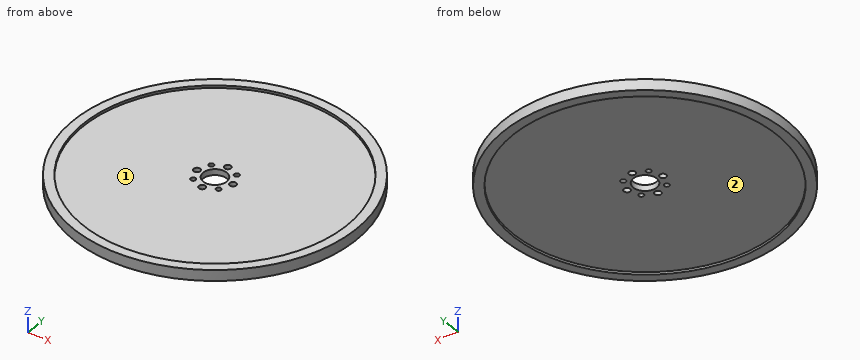
from build123d import *

# Parameters (mm, degrees)
SKETCH1_R                 = 76.2
SKETCH1_R_2               = 71.12
BOSS_EXTRUDE1_DEPTH       = 2.921
SKETCH3_R                 = 71.12
SKETCH3_R_2               = 6.35
SKETCH3_R_3               = 1.778
BOSS_EXTRUDE2_DEPTH       = 1.5875
F_6_32_TAPPED_HOLE1_D     = 2.7051
F_6_32_TAPPED_HOLE1_DEPTH = 3.175


with BuildPart() as part:
    # Sketch1 → Boss-Extrude1 (new body, symmetric)
    with BuildSketch(Plane.XY):
        Circle(SKETCH1_R)
        Circle(SKETCH1_R_2, mode=Mode.SUBTRACT)
    extrude(amount=BOSS_EXTRUDE1_DEPTH, both=True)

    # Sketch3 → Boss-Extrude2 (add, symmetric)
    with BuildSketch(Plane.XY):
        Circle(SKETCH3_R)
        Circle(SKETCH3_R_2, mode=Mode.SUBTRACT)
        with Locations((0, 9.779)):
            Circle(SKETCH3_R_3, mode=Mode.SUBTRACT)
        with Locations((9.779, 0)):
            Circle(SKETCH3_R_3, mode=Mode.SUBTRACT)
        with Locations((0, -9.779)):
            Circle(SKETCH3_R_3, mode=Mode.SUBTRACT)
        with Locations((-9.779, 0)):
            Circle(SKETCH3_R_3, mode=Mode.SUBTRACT)
    extrude(amount=BOSS_EXTRUDE2_DEPTH, both=True)

    # #6-32 Tapped Hole1
    with Locations(Plane.XY.offset(1.5875)):
        with Locations((-6.914797213, 6.914797213), (6.914797213, 6.914797213), (6.914797213, -6.914797213), (-6.914797213, -6.914797213)):
            Hole(F_6_32_TAPPED_HOLE1_D / 2, depth=F_6_32_TAPPED_HOLE1_DEPTH)


solid = part.part
For this review, take the finished solid that the model builds, in its own axes (mm). Face numbers are marked on the shaded views. A direction names the side the tool comes from. Give positions to 0.01 mm unless a question says otherwise; leave off trailing zeros. Loops run counter-clockwise (first coordinate to the right, second up) from the corner with the lowest first, then second, coordinate; pieces in that order, holes last. Notation, with made-up numbers: M -7,29 L 0,29 A26 ccw 0,54 Z; hole C -14,36.25 d1. An arc over 180 degrees is marked long. Put each result on its own line as item: value. Start each with the question number.
(1) For pin 1 (3.5 mm diameter, centred on x = 6.91, y = 6.91, fed in from +Z); pin 2 (3 mm diameter, centred on x = -6.91, y = 6.91, fed in from -Z); pin 3 (3 mm diameter, centred on x = 0, y = 9.779, fed in from -Z); pin 4 (1 mm diameter, centred on y = 24, z = -1.5, fed in from +X), all flat-tipped, find the tip position at first contact; note any pin that passes through.
(2) Wall thickness on L1, parallel to Y at x = 0, z = -0.35; L2, parallel to Y at x = 0, z = -2.4; L3, parallel to Z at x = -32, y = 18: over which ranges is each line inside the solid? List them lowest first.
(3) Machinability: for the marked faces 1 and 2, which of the approach directions +Z, -Z, +X, -X, +Y, -Y give a long, thin tool a straight path to every point of the face, cutting with its end or side? Answer none if there is none.
(4) Add section D-D, the plane x = 25.5. Write out the cut boundary in (y, z), then the cut area to 3 significant figures.
(5) Add section C-C, the plane z = -0.7. Give the number of separate pieces and of enclosed holes in the cut face, then the cut area to 3 significant figures.
(6) Add section A-A, the plane x = 0. Write out the cut boundary in (y, z), then the cut area to 3 significant figures.
Result:
1. pin 1: stops at z = 1.59
1. pin 2: stops at z = -1.59
1. pin 3: passes through
1. pin 4: stops at x = 72.49
2. L1: y = -76.2 to -11.56, -8 to -6.35, 6.35 to 8, 11.56 to 76.2
2. L2: y = -76.2 to -71.12, 71.12 to 76.2
2. L3: z = -1.59 to 1.59
3. face 1: +Z
3. face 2: -Z
4. outline: M -71.81,-2.92 L -66.39,-2.92 L -66.39,-1.59 L 66.39,-1.59 L 66.39,-2.92 L 71.81,-2.92 L 71.81,2.92 L 66.39,2.92 L 66.39,1.59 L -66.39,1.59 L -66.39,2.92 L -71.81,2.92 Z
4. area: 485 mm^2
5. separate pieces: 1
5. enclosed holes: 9
5. area: 18,100 mm^2
6. outline: M -76.2,-2.92 L -71.12,-2.92 L -71.12,-1.59 L -11.56,-1.59 L -11.56,1.59 L -71.12,1.59 L -71.12,2.92 L -76.2,2.92 Z; M -8,-1.59 L -6.35,-1.59 L -6.35,1.59 L -8,1.59 Z; M 6.35,-1.59 L 8,-1.59 L 8,1.59 L 6.35,1.59 Z; M 11.56,-1.59 L 71.12,-1.59 L 71.12,-2.92 L 76.2,-2.92 L 76.2,2.92 L 71.12,2.92 L 71.12,1.59 L 11.56,1.59 Z
6. area: 448 mm^2
